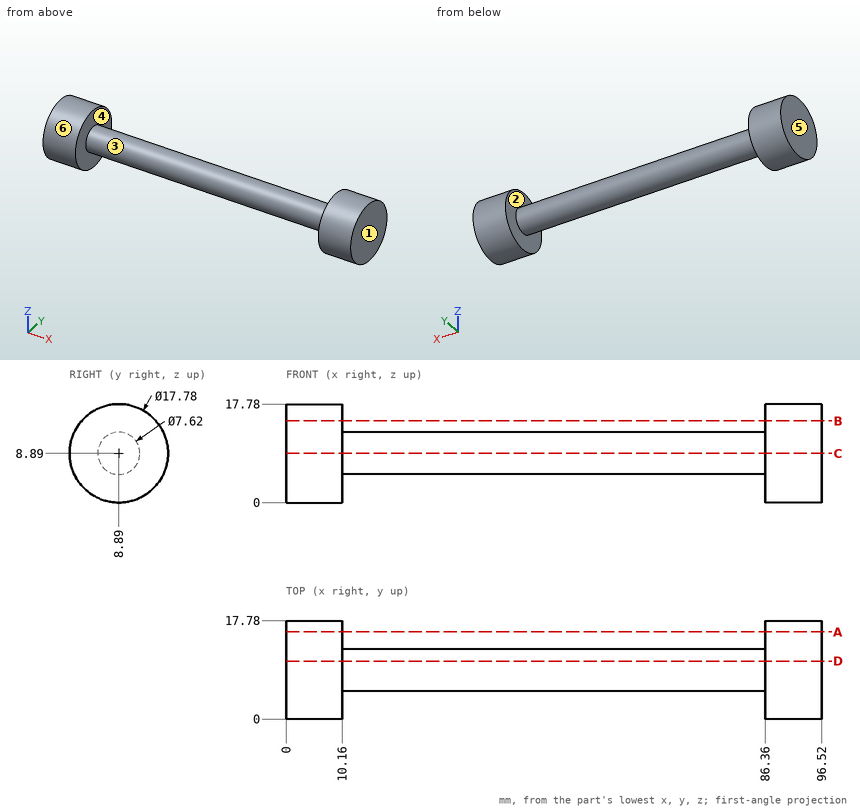
Design review of the part shown in the three views and the two pictorial views. Dimensions are in mm from the part's minimum x, y and z. A direction names the side the tool comes from. Coordinates: 2 decimals unless noted, no trailing zeros. Write each loop counter-clockwise with the first axis right and the second up, starting at its lowest first coordinate (ties: lowest second). Pieces come first, ordered by that corner, then holes.
(1) The part is to be moulded in two halves that separate along X. For the marked faces 3, 4, 5 and 6, say which applies: +X half, -X half, draft (parallel to the pull), parting line (faces both ways), or undercut.
(2) For pin 1 Ø6 at (x, y) = (38.5, 10.5) entering from -Z; pin 2 Ø8 at (y, z) = (14.5, 10) entering from -X; pin 3 Ø1 at (x, y) = (22.5, 6) entering from -Z, all flat-tipped, find the tip position at first contact; note any pin that passes through.
(3) Wall thickness on probe 1 along X at (y, z) = (6.75, 16); probe 2 along Z at (x, y) = (17.5, 9.25); probe 3 along Y at (x, z) = (14, 9): over which ranges is each line inside the solid? List them lowest first.
(4) Add section A-A on y = 15.75. Give the boundary of the cut face in (x, z), then the cut area to 3 significant figures.
(5) Add section D-D on y = 10.5. Give the boundary of the cut face in (x, z).
(6) Add section B-B on z = 14.75. Give the boundary of the cut face in (x, y), then the cut area to 3 significant figures.
(7) Tool access review of the marked faces 1 and 2: name each direction out of +Z, -Z, +X, -X, +Y, -Y from which nothing blocks a thin tool from reaching the whole face with its end or side.
(8) Add section C-C on z = 8.89. Give the boundary of the cut face in (x, y).
Answer sheet:
1. face 3: undercut
1. face 4: undercut
1. face 5: -X half
1. face 6: draft
2. pin 1: stops at z = 5.08
2. pin 2: stops at x = 0
2. pin 3: stops at z = 5.92
3. probe 1: x = 0 to 10.16, 86.36 to 96.52
3. probe 2: z = 5.1 to 12.68
3. probe 3: y = 5.08 to 12.7
4. outline: (0, 3.24) - (10.16, 3.24) - (10.16, 14.54) - (0, 14.54) - close; (86.36, 3.24) - (96.52, 3.24) - (96.52, 14.54) - (86.36, 14.54) - close
4. area: 230 mm2
5. outline: (0, 0.15) - (10.16, 0.15) - (10.16, 5.44) - (86.36, 5.44) - (86.36, 0.15) - (96.52, 0.15) - (96.52, 17.63) - (86.36, 17.63) - (86.36, 12.34) - (10.16, 12.34) - (10.16, 17.63) - (0, 17.63) - close
6. outline: (0, 2.2) - (10.16, 2.2) - (10.16, 15.58) - (0, 15.58) - close; (86.36, 2.2) - (96.52, 2.2) - (96.52, 15.58) - (86.36, 15.58) - close
6. area: 272 mm2
7. face 1: +Z, -Z, +X, +Y, -Y
7. face 2: none
8. outline: (0, 0) - (10.16, 0) - (10.16, 5.08) - (86.36, 5.08) - (86.36, 0) - (96.52, 0) - (96.52, 17.78) - (86.36, 17.78) - (86.36, 12.7) - (10.16, 12.7) - (10.16, 17.78) - (0, 17.78) - close
